Work out the finished part from the listing and answer in its coordinate system (mm). A direction names the side the tool comes from. Round coordinates to 2 decimals unless told otherwise and drop trailing zeros. Write each loop counter-clockwise with the first axis right and the second up, starting at its lowest first coordinate (ties: lowest second). Pieces come first, ordered by that corner, then holes.
1. A tool of negligible diameter and unlimited length cuts with its end or side. For faces 1 (the face through (4, 0, -6.928)), 2 (the face through (17, 4, 4)), 3 (the face through (27, -3, -3)), from which of +Z, -Z, +X, -X, +Y, -Y can it reach the whole face along a straight path? Write none if from no direction.
2. Flat-ended cylindrical pins translate along their axes: pin 1 Ø8 at (x, z) = (-20, 6) entering from -Y; pin 2 Ø2.5 at (y, z) = (-1, -1) entering from -X; pin 3 Ø1.3 at (y, z) = (-4, -5.5) entering from +X; pin 4 Ø6 at (x, z) = (-19, 4.5) entering from -Y. Find the tip coordinate at first contact, or state that the pin passes through.
3. Find section A-A (x = 5). Write down the section's boundary in (y, z), and give its area (3 significant figures).
4. Determine the mould class of faces 4 (the face through (21.44, -5.11, -0.22)), 5 (the face through (8, 7.2, -0.2)), 6 (the face through (13.8, -0.41, -3.09)) for opening direction Y: pulls with the +Y half, pulls with the -Y half, needs draft (parallel to the pull), parting line crosses it, or undercut.
5. Find section B-B (x = -18.5). Write down the section's boundary in (y, z).
6. Straight lines are drawn through the part: probe 1 along Z at (x, y) = (-15.75, 0); probe 2 along X at (y, z) = (2, -4); probe 3 along X at (y, z) = (-2.5, 6.75). For each, find the intervals that lie inside material, in ascending order.
Autodesk Inventor part; units mm, degrees
ref_plane "YZ Plane" through (0, 0, 0) normal (1, 0, 0) x (0, 1, 0)
ref_plane "XZ Plane" through (0, 0, 0) normal (0, 1, 0) x (-1, 0, 0)
ref_plane "XY Plane" through (0, 0, 0) normal (0, 0, 1) x (1, 0, 0)
sketch "Sketch1" plane through (0, 0, 0) normal (0, 0, 1) x (1, 0, 0)
  line L0 (-20, 4.75) -> (-20, 5.7007)
  line L1 (-20, 5.7007) -> (-25, 4.75)
  line L2 (-20, 4.75) -> (-15, 4.75)
  line L3 (-10, 6.0299) -> (-15, 4.75)
  line L4 (-10, 5.3899) -> (0, 5.3899)
  line L5 (-10, 6.0299) -> (-10, 5.3899)
  line L6 (-27.5, 4.75) -> (-27.5, 4)
  line L7 (-27.5, 4.75) -> (-25, 4.75)
  line L8 (-27.5, 4) -> (0, 4)
  line L9 (0, 8) -> (8, 8)
  line L10 (0, 8) -> (0, 5.3899)
  line L11 (8, 8) -> (8, 7)
  line L12 (8, 7) -> (9, 7)
  line L13 (9, 9) -> (17, 9)
  line L14 (26, 3.1165) -> (0, 3.1165)
  line L15 (0, 4) -> (0, 3.1165)
  line L16 (9, 9) -> (9, 7)
  line L17 (26, 4) -> (26, 5.1165)
  line L18 (26, 5.1165) -> (17, 5.1165)
  line L19 (17, 5.1165) -> (17, 9)
  line L20 (26, 4) -> (27, 4)
  line L21 (27, 4) -> (27, 5.1165)
  line L22 (27, 5.1165) -> (28, 5.1165)
  line L23 (28, 5.1165) -> (28, 3.1165)
  line L24 (28, 3.1165) -> (26, 3.1165)
  line L25 (-35.0249, 0) -> (33.4829, 0)
  point P0 (0, 0)
  point P1 (0, 4.75)
  point P2 (13, 7)
  dimension "d3" = 5
  dimension "d4" = 5
  dimension "d14" = 0.75
  dimension "d15" = 1
  dimension "d16" = 8
  dimension "d26" = 2
  dimension "d27" = 1
  dimension "d28" = 1
sketch "Sketch2" plane through (0, 0, 0) normal (0, 0, 1) x (1, 0, 0)
  point P0 (0, 0)
sketch "Sketch3" plane through (0, 0, 0) normal (0, 0, 1) x (1, 0, 0)
  point P0 (0, 0)
sketch "Sketch4" plane through (0, 0, 0) normal (0, 0, 1) x (1, 0, 0)
  point P0 (0, 0)
sketch "Sketch5" plane through (0, 0, 0) normal (1, 0, 0) x (0, 1, 0)
  point P0 (0, 0)
sketch "Sketch6" plane through (0, 0, 0) normal (0, 0, 1) x (1, 0, 0)
  line L0 (8.9873, 9.0104) -> (8.9873, 6.9688)
  point P0 (0, 0)
sketch "Sketch7" plane through (0, 0, 0) normal (0, 0, 1) x (1, 0, 0)
  point P0 (0, 0)
sketch "Sketch8" plane through (0, 0, 0) normal (0, 0, 1) x (1, 0, 0)
  point P0 (0, 0)
revolve "Revolution1" add sketch "Sketch1" angle 360 about axis through (-35.0249, 0, 0) along (1, 0, 0)
sketch "Sketch9" plane through (17, 0, 0) normal (1, 0, 0) x (0, 0, -1)
  circle A0 centre (0, 0) radius 7
  circle A1 centre (0, 0) radius 9
  circle A2 centre (0, 0) radius 9
  circle A3 centre (0, 0) radius 5.1165
  circle A4 centre (0, 0) radius 3.1165
  circle A5 centre (0, 0) radius 5.7007
  line L0 (0, 9) -> (7.7942, 4.5)
  line L1 (7.7942, 4.5) -> (7.7942, -4.5)
  line L2 (7.7942, -4.5) -> (0, -9)
  line L3 (0, -9) -> (-7.7942, -4.5)
  line L4 (-7.7942, -4.5) -> (-7.7942, 4.5)
  line L5 (-7.7942, 4.5) -> (0, 9)
  point P0 (0, -9)
  point P1 (0, -9)
  point P2 (7.7942, -4.5)
  point P3 (7.7942, -4.5)
extrude "Extrusion1" cut sketch "Sketch9" against normal blind 8 contours A1 L1 | L0 A1 | A1 L2 | L5 A1 | A1 L3 | L4 A1
sketch "Sketch10" plane through (0, 0, 0) normal (-1, 0, 0) x (0, 0, 1)
  circle A0 centre (0, 0) radius 5.3899
  circle A1 centre (0, 0) radius 8
  circle A2 centre (0, 0) radius 3.1165
  circle A3 centre (0, 0) radius 4
  circle A4 centre (0, 0) radius 5.3899
  circle A5 centre (0, 0) radius 8
  circle A6 centre (0, 0) radius 3.1165
  circle A7 centre (0, 0) radius 4
  circle A8 centre (0, 0) radius 8
  line L0 (6.9282, -4) -> (0, -8)
  line L1 (0, -8) -> (-6.9282, -4)
  line L2 (-6.9282, -4) -> (-6.9282, 4)
  line L3 (-6.9282, 4) -> (0, 8)
  line L4 (0, 8) -> (6.9282, 4)
  line L5 (6.9282, 4) -> (6.9282, -4)
  point P0 (0, 8)
  point P1 (0, 8)
  point P2 (-6.9282, 4)
  point P3 (-6.9282, 4)
  point P4 (0, -8)
  point P5 (0, -8)
extrude "Extrusion2" cut sketch "Sketch10" against normal blind 8 contours A1 L5 | L4 A1 | A1 L0 | L3 A1 | A1 L1 | L2 A1
chamfer "Chamfer1" distance 0.2 angle 45 1 edges at (-20, -5.7007, 0)
chamfer "Chamfer2" distance 0.2 angle 45 1 edges at (-10, -6.0299, 0)
properties part number "sambungan cilek ng gede"
Worked answers:
1. face 1: -Z, -X, +Y, -Y
1. face 2: +X
1. face 3: none
2. pin 1: stops at y = -5.3
2. pin 2: passes through
2. pin 3: stops at x = 17
2. pin 4: stops at y = -5.39
3. outline: (-8, 0) - (-4, -6.93) - (4, -6.93) - (8, 0) - (4, 6.93) - (-4, 6.93) - close; hole circle Ø6.23 at (0, 0)
3. area: 136 mm2
4. face 4: parting line crosses it
4. face 5: needs draft
4. face 6: undercut
5. outline: circle Ø9.5 at (0, 0); hole circle Ø8 at (0, 0)
6. probe 1: z = -4.75 to -4, 4 to 4.75
6. probe 2: x = -27.5 to 26, 27 to 28
6. probe 3: x = 0 to 8, 9 to 17
